The listing builds one solid part. Answer for the finished solid, in the listing's coordinates (mm). Face numbers are marked on the shaded views. A direction names the side the tool comes from. Give positions to 0.01 mm unless a question says otherwise; leave off trailing zeros. Write each loop counter-clockwise with the first axis right and the second up, starting at its lowest first coordinate (ties: lowest second). Pieces come first, ordered by that corner, then holes. Notation, with made-up numbers: M 56.25,70 L 113.25,70 A27 ccw 113.25,88 Z; hole C 38.5,55.25 d1. An arc over 180 degrees is marked long. Return JSON: item names as keys, results as strings.
from build123d import *

# Parameters (mm, degrees)
SZKIC2_R                   = 0.5
WYTNIJ_WYCI_GNI_CIE1_DEPTH = 1


with BuildPart() as part:
    # Szkic1 → Obrót1 (revolve)
    with BuildSketch(Plane.XY, mode=Mode.PRIVATE) as obr_t1_sk:
        Polygon((-6, 12.5), (6, 12.5), (6, 18), (12, 18), (12, 16), (9, 16), (9, 10.5), (12.5, 10.5), (12.5, 7.5), (-12.5, 7.5), (-12.5, 10.5), (-9, 10.5), (-9, 16), (-12, 16), (-12, 18), (-6, 18), align=None)
    revolve(obr_t1_sk.sketch.rotate(Axis((-30.837457467, 0, 0), (1, 0, 0)), 90), axis=Axis((-30.837457467, 0, 0), (1, 0, 0)))

    # Szkic2 → Wytnij-wyciągnięcie1 (cut)
    with BuildSketch(Plane.ZY.offset(12)):
        with Locations((0, 17)):
            Circle(SZKIC2_R)
    extrude(amount=-WYTNIJ_WYCI_GNI_CIE1_DEPTH, mode=Mode.SUBTRACT)


solid = part.part
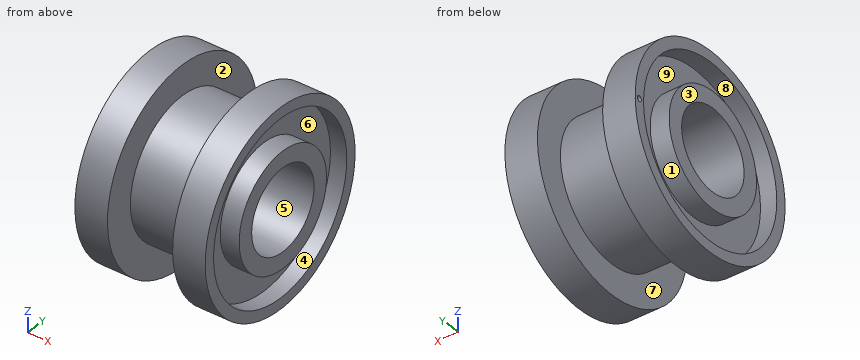
Item 1: Which of the six approach directions +Z, -Z, +X, -X, +Y, -Y give full straight-line access (tool end or side, diameter ignored) to the marked faces 1, 2, 3, 4 and 5?
Geometry results:
{"face 1": "-X", "face 2": "none", "face 3": "+Z, -Z, -X, +Y, -Y", "face 4": "+X", "face 5": "+X, -X"}
Item 2: Given pin 1 Ø8 at (x, y) = (-8.5, -10.5) entering from -Z; pin 2 Ø12 at (x, z) = (-7.5, -3.5) entering from -Y; pin 3 Ø1.5 at (x, z) = (4, -8) entering from +Y, each flat-ended and moving along its own axis, determine where each tip first touches the part or whether it passes through.
Geometry results:
{"pin 1": "stops at z = -16.79", "pin 2": "stops at y = -18", "pin 3": "stops at y = 10.18"}
Item 3: Determine the mould class of the marked faces 6, 7, 8 and 9 for opening direction X: +X half, -X half, draft (parallel to the pull), parting line (faces both ways), or undercut.
Geometry results:
{"face 6": "+X half", "face 7": "undercut", "face 8": "draft", "face 9": "-X half"}
Item 4: Find the intervals of material crossed by line 1 (Y direction, x = -11.4, z = 0); line 2 (Y direction, x = -10.95, z = 0); line 3 (X direction, y = 12.5, z = 5), in increasing order.
Geometry results:
{"line 1": "y = -18 to -16, -10.5 to -7.5, 7.5 to 10.5, 16 to 16.5, 17.5 to 18", "line 2": "y = -18 to -16, -10.5 to -7.5, 7.5 to 10.5, 16 to 18", "line 3": "x = -9 to -6, 6 to 9"}
Item 5: A cutting plane is placed at D-D, the plane y = 11. Write down the section's boundary in (x, z).
Geometry results:
{"outline": "M -12,-14.25 L -6,-14.25 L -6,-5.94 L 6,-5.94 L 6,-14.25 L 12,-14.25 L 12,-11.62 L 9,-11.62 L 9,11.62 L 12,11.62 L 12,14.25 L 6,14.25 L 6,5.94 L -6,5.94 L -6,14.25 L -12,14.25 L -12,11.62 L -9,11.62 L -9,-11.62 L -12,-11.62 Z"}
Item 6: A cutting plane is placed at C-C, the plane x = -2. Write down the section's boundary in (y, z).
Geometry results:
{"outline": "C 0,0 d25; hole C 0,0 d15"}
